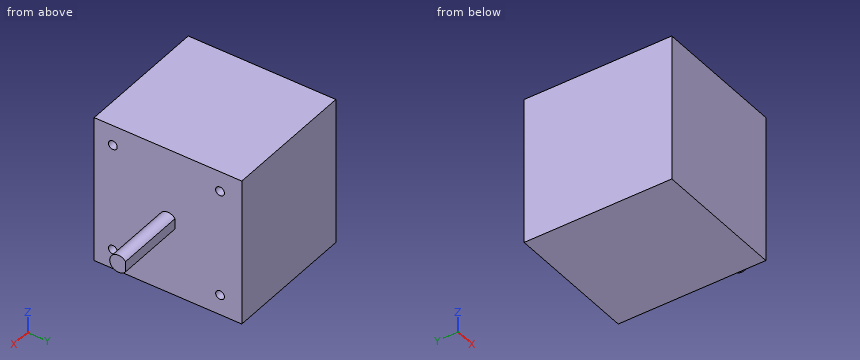
from build123d import *

# Parameters (mm, degrees)
SKETCH_1_W          = 42
SKETCH_1_H          = 42
EXTRUDE_1_DEPTH     = 38
EXTRUDE_2_DEPTH     = 20
SKETCH_3_R          = 1.25
CUT_EXTRUDE_1_DEPTH = 20


with BuildPart() as part:
    # 草图1 → 凸台-拉伸1 (new body)
    with BuildSketch(Plane(origin=(0, 0, 0), x_dir=(0, 0, -1), z_dir=(1, 0, 0))):
        Rectangle(SKETCH_1_W, SKETCH_1_H)
    extrude(amount=EXTRUDE_1_DEPTH)

    # 草图2 → 凸台-拉伸2 (add)
    with BuildSketch(Plane(origin=(38, 0, 0), x_dir=(0, 0, -1), z_dir=(1, 0, 0))):
        with BuildLine():
            Line((-1.5, 2), (1.5, 2))
            ThreePointArc((1.5, 2), (0, -2.5), (-1.5, 2))
        make_face()
    extrude(amount=EXTRUDE_2_DEPTH)

    # 草图3 → 切除-拉伸1 (cut)
    with BuildSketch(Plane(origin=(38, 0, 0), x_dir=(0, 0, -1), z_dir=(1, 0, 0))):
        with Locations((-15.25, 14.812372141)):
            Circle(SKETCH_3_R)
        with Locations((15.25, 14.812372141)):
            Circle(SKETCH_3_R)
        with Locations((15.476779335, -15.687627859)):
            Circle(SKETCH_3_R)
        with Locations((-15.25, -15.687627859)):
            Circle(SKETCH_3_R)
    extrude(amount=-CUT_EXTRUDE_1_DEPTH, mode=Mode.SUBTRACT)


solid = part.part
Here's how the part is built. I have some questions about the finished solid (model axes, mm). Round coordinates to 2 decimals unless told otherwise and drop trailing zeros. Write each loop counter-clockwise with the first axis right and the second up, starting at its lowest first coordinate (ties: lowest second). Pieces come first, ordered by that corner, then holes. Notation, with made-up numbers: (-26, -37.5) -> (26, -37.5) arc R31 cw to (26, 1.5) -> close; hole circle Ø6 at (-31.5, 59). An arc over 180 degrees is marked (long way). One line per item, written item: value.
1) Suppose I cut it at A-A on z = 0. List the corners of the cut face in (x, y) for me.
Filled sheet:
outline: (0, -21) -> (38, -21) -> (38, -2.5) -> (58, -2.5) -> (58, 2) -> (38, 2) -> (38, 21) -> (0, 21) -> close
2) Suppose I cut it at B-B on y = 0.5. List the corners of the cut face in (x, z) for me, plus the area to 3 significant figures.
Filled sheet:
outline: (0, -21) -> (38, -21) -> (38, -2.45) -> (58, -2.45) -> (58, 2.45) -> (38, 2.45) -> (38, 21) -> (0, 21) -> close
area: 1,690 mm2
3) I'm going to push flat-ended pins straight in: pin 1 Ø3 at (y, z) = (14.81, -15.25) entering from +X; pin 2 Ø1.5 at (x, z) = (47.5, 0.5) entering from +Y; pin 3 Ø1.2 at (y, z) = (14.5, -15) entering from +X. Where does each tip first touch, or does it pass through?
Filled sheet:
pin 1: stops at x = 38
pin 2: stops at y = 2
pin 3: stops at x = 18
4) Suppose I cut it at D-D on z = 15.25. List the corners of the cut face in (x, y) for me, plus the area to 3 significant figures.
Filled sheet:
outline: (0, -21) -> (38, -21) -> (38, -16.94) -> (18, -16.94) -> (18, -14.44) -> (38, -14.44) -> (38, 13.56) -> (18, 13.56) -> (18, 16.06) -> (38, 16.06) -> (38, 21) -> (0, 21) -> close
area: 1,500 mm2
5) Suppose I cut it at C-C on x = 40.5. List the corners of the cut face in (y, z) for me, plus the area to 3 significant figures.
Filled sheet:
outline: (2, -1.5) -> (2, 1.5) arc R2.5 ccw (long way) to start
area: 18.6 mm2
6) If I drill on line 1 (Y direction, x = 30, z = 15.25); line 2 (X direction, y = 17, z = -14); line 3 (Y direction, x = 26, z = 15), over which ranges is the centre line in solid material (lowest first)? Write a range as [from, to].
Filled sheet:
line 1: y = [-21, -16.94], [-14.44, 13.56], [16.06, 21]
line 2: x = [0, 38]
line 3: y = [-21, -16.91], [-14.46, 13.59], [16.04, 21]
